Geometry check sheet. Reference: the model listing, model coordinates, mm. Round coordinates to 2 decimals unless told otherwise and drop trailing zeros. Write each loop counter-clockwise with the first axis right and the second up, starting at its lowest first coordinate (ties: lowest second). Pieces come first, ordered by that corner, then holes.
Item 1: Depth check by flat-ended pin: P1, Ø1.5, axis at y = -6, z = 5.5, coming from the -X side; P2, Ø1.5, axis at x = 9.5, y = -2, coming from the -Z side; P3, Ø4, axis at x = -8.5, y = -2.5, coming from the +Z side; P4, Ø3, axis at x = -13, y = -5.5, coming from the +Z side. Enter the tip coordinate at first touch or a pass-through.
Item 2: Scan lines: probe 1 along Z at (x, y) = (7, 11.5); probe 2 along X at (y, z) = (16, 2.5); probe 3 along Y at (x, z) = (2, 32). Record each from-to range of solid material in increasing order.
Item 3: Cross-section at A-A (z = 17). Enter the section's corners in (x, y).
Item 4: Cross-section at B-B (z = 31.5). Enter the section's corners in (x, y).
from build123d import *

# Parameters (mm, degrees)
F2_R = 5.08
F3_R = 0.635


with BuildPart() as f1:
    # F0 (on Front) → F1 (revolve)
    with BuildSketch(Plane.XZ):
        with BuildLine():
            ThreePointArc((-3.768967, 7.97639), (-4.492542, 6.243991), (-6.208299, 5.481795))
            Line((-6.208299, 5.481795), (-16.375725, 5.08))
            Line((-16.375725, 5.08), (-19.05, 0))
            Line((-19.05, 0), (0, 0))
            Line((0, 0), (0, 42.714926))
            Line((0, 42.714926), (-3.175, 42.714926))
            ThreePointArc((-3.175, 42.714926), (-2.256928, 25.324883), (-3.768967, 7.97639))
        make_face()
    revolve(axis=Axis((0, 0, 25.4), (0, 0, 1)))

    # F2
    f2_edges = [f1.edges().sort_by_distance(p)[0] for p in [
        (16.375725, 0, 5.08),
    ]]
    fillet(f2_edges, radius=F2_R)

    # F3
    f3_edges = [f1.edges().sort_by_distance(p)[0] for p in [
        (19.05, 0, 0),
    ]]
    fillet(f3_edges, radius=F3_R)


solid = f1.part
Resolved:
1. P1: stops at x = -14.14
1. P2: stops at z = 0
1. P3: stops at z = 5.46
1. P4: stops at z = 5.23
2. probe 1: z = 0 to 5.2
2. probe 2: x = -7.65 to 7.65
2. probe 3: y = -1.18 to 1.18
3. outline: circle Ø5.36 at (0, 0)
4. outline: circle Ø4.61 at (0, 0)
